Autodesk Inventor part; units mm, degrees
ref_plane "YZ Plane" through (0, 0, 0) normal (1, 0, 0) x (0, 1, 0)
ref_plane "XZ Plane" through (0, 0, 0) normal (0, 1, 0) x (-1, 0, 0)
ref_plane "XY Plane" through (0, 0, 0) normal (0, 0, 1) x (1, 0, 0)
sketch "Sketch1" plane through (0, 0, 0) normal (0, 1, 0) x (-1, 0, 0)
  line L0 (0, 4.5) -> (-12.7, 4.5)
  line L1 (-12.7, 4.5) -> (-12.7, -4.5)
  line L2 (-12.7, -4.5) -> (0, -4.5)
  line L3 (0, 4.5) -> (0.254, 4.5)
  line L4 (0.254, -4.5) -> (0, -4.5)
  line L5 (6.35, 4.5) -> (6.35, -4.5)
  line L6 (6.35, 7.548) -> (6.35, 4.5)
  line L7 (6.35, -7.548) -> (6.35, -4.5)
  line L8 (0.254, 4.5) -> (6.35, 7.548)
  line L9 (0.254, -4.5) -> (6.35, -7.548)
  point P0 (0, 0)
  point P1 (0, -4.5)
  dimension "d1" = 9
  dimension "d2" = 4.5
  dimension "d7" = 3.048
  dimension "d8" = 3.048
  dimension "d9" = 12.954
  dimension "d16" = 6.096
extrude "Shape" add sketch "Sketch1" along normal blind 25.4
sketch "Sketch2" plane through (-0.254, 0, 4.5) normal (0, 0, 1) x (1, 0, 0)
  line L0 (4.7625, 19.05) -> (9.5125, 19.05)
  line L1 (9.5125, 19.05) -> (9.5125, 6.35)
  line L2 (9.5125, 6.35) -> (4.7625, 6.35)
  line L3 (4.7625, 6.35) -> (4.7625, 19.05)
  point P0 (0.254, 0)
  dimension "d12" = 4.75
  dimension "d13" = 12.7
extrude "Bridge" cut sketch "Sketch2" against normal through all
sketch "Sketch3" plane through (4.5085, 6.35, 4.5) normal (1, 0, 0) x (0, 0, -1)
  line L0 (9, 12.7) -> (9, 0) construction
  line L1 (0, 12.7) -> (9, 12.7) construction
  line L2 (9, 0) -> (0, 0) construction
  line L3 (0, -6.35) -> (0, 19.05)
  line L4 (9, -6.35) -> (9, 19.05)
  line L5 (0, 9.7549) -> (9, 9.7549)
  line L6 (9, 9.7549) -> (9, 9.6279)
  line L7 (9, 9.6279) -> (0, 9.6279)
  line L8 (0, 9.6279) -> (0, 9.7549)
  line L9 (0, 6.35) -> (9, 6.35)
  line L10 (9, 6.35) -> (9, 6.223)
  line L11 (9, 6.223) -> (0, 6.223)
  line L12 (0, 6.223) -> (0, 6.35)
  line L13 (0, 3.175) -> (9, 3.175)
  line L14 (9, 3.175) -> (9, 3.048)
  line L15 (9, 3.048) -> (0, 3.048)
  line L16 (0, 3.048) -> (0, 3.175)
  point P0 (4.5, -6.35)
  point P1 (0, 3.048)
  point P2 (0, 6.223)
  point P3 (9, 6.35)
  point P4 (0, 9.6279)
  point P5 (9, 9.7549)
  dimension "d17" = 0.127
  dimension "d18" = 0.127
  dimension "d19" = 0.127
  dimension "d20" = 2.9451
  dimension "d22" = 9.525
extrude "Supports" add sketch "Sketch3" along normal up to surface (4.75 mm away) contours L3 L13 L4 L15 | L3 L9 L4 L11 | L3 L5 L4 L7
equation "\"d8\" = d7"
equation "\"d18\" = d17"
equation "\"d19\" = d17"
properties part number "Sliding test insert"
Verification items for the finished model (mm, model axes). A direction names the side the tool comes from. Round coordinates to 2 decimals unless told otherwise and drop trailing zeros. Write each loop counter-clockwise with the first axis right and the second up, starting at its lowest first coordinate (ties: lowest second). Pieces come first, ordered by that corner, then holes. Notation, with made-up numbers: (81, -26.5) - (93, -26.5) arc R13 cw to (93, -19.5) - close; hole circle Ø3 at (83, -0.5). An arc over 180 degrees is marked (long way). Answer as a JSON object with one key per item and string values. Group by question number.
Q1. Mould release check, pull along Y, two halves, no side actions. Record for faces 1 (the flat face through (4.508, 14, 0)), 2 (the flat face through (3, 25.4, 0)), 3 (the flat face through (3, 0, 0)), 4 (the flat face through (-6.35, 13, 0)): released by +Y, released by -Y, zero draft, split by the parting line, or undercut.
Q2. Tool access check on faces 5 (the flat face through (9.258, 18, 0)), 6 (the flat face through (12.7, 13, 0)), 7 (the flat face through (3, 13, 4.5)), 8 (the flat face through (3, 13, -4.5)). Record the directions out of +Z, -Z, +X, -X, +Y, -Y that give a thin tool (end or side, any length) a straight path to the whole face; none if there is none.
Q3. Section check B-B, the plane y = 15.5. Enter the section's corners in (x, z), plus the area to 3 significant figures.
Q4. Thickness scan on line 1 (X direction, y = 8, z = 0.25); line 2 (Z direction, x = 1, y = 3.75); line 3 (X direction, y = 3.25, z = 5.5). Record the ranges inside material, lowest first.
Q5. Section check C-C, the plane z = 3.5. Give the number of separate pieces and of enclosed holes in the cut face, plus the area to 3 significant figures.
Q6. Section check D-D, the plane y = 20.5. Enter the section's corners in (x, z).
Q7. Go/stop test with flat-tipped pins: pin 1 Ø5 at (x, y) = (0, 13.5) entering from -Z; pin 2 Ø6 at (x, y) = (2, 16) entering from +Z; pin 3 Ø4 at (x, y) = (9.5, 3.5) entering from +Z. Record where each tip stops, or that it passes through.
Q8. Section check A-A, the plane x = 8.75. Enter the section's corners in (y, z) (3 decimals), plus the area to 3 significant figures.
Found:
{
 "1": {"face 1": "undercut", "face 2": "released by +Y", "face 3": "released by -Y", "face 4": "zero draft"},
 "2": {"face 5": "+Z, -Z", "face 6": "+Z, -Z, +X, +Y, -Y", "face 7": "+Z, +X, +Y, -Y", "face 8": "-Z, +X, +Y, -Y"},
 "3": {"outline": "(-6.35, -7.55) - (-0.25, -4.5) - (4.51, -4.5) - (4.51, 4.5) - (-0.25, 4.5) - (-6.35, 7.55) - close; (9.26, -4.5) - (12.7, -4.5) - (12.7, 4.5) - (9.26, 4.5) - close", "area": "147 mm^2"},
 "4": {"line 1": "x = -6.35 to 4.51, 9.26 to 12.7", "line 2": "z = -4.5 to 4.5", "line 3": "x = -6.35 to -2.25"},
 "5": {"separate pieces": "1", "enclosed holes": "4", "area": "425 mm^2"},
 "6": {"outline": "(-6.35, -7.55) - (-0.25, -4.5) - (12.7, -4.5) - (12.7, 4.5) - (-0.25, 4.5) - (-6.35, 7.55) - close"},
 "7": {"pin 1": "stops at z = -5.62", "pin 2": "stops at z = 4.87", "pin 3": "stops at z = 4.5"},
 "8": {"outline": "(0, -4.5) - (6.35, -4.5) - (6.35, 4.5) - (0, 4.5) - close; (9.398, -4.5) - (9.525, -4.5) - (9.525, 4.5) - (9.398, 4.5) - close; (12.573, -4.5) - (12.7, -4.5) - (12.7, 4.5) - (12.573, 4.5) - close; (15.978, -4.5) - (16.105, -4.5) - (16.105, 4.5) - (15.978, 4.5) - close; (19.05, -4.5) - (25.4, -4.5) - (25.4, 4.5) - (19.05, 4.5) - close", "area": "118 mm^2"}
}
